Geometry: final body of the model. Coordinates: model frame, mm. A direction names the side the tool comes from. Coordinates: 2 decimals unless noted, no trailing zeros. Write each loop counter-clockwise with the first axis right and the second up, starting at its lowest first coordinate (ties: lowest second). Pieces come first, ordered by that corner, then holes.
from build123d import *

# Parameters (mm, degrees)
SKETCH1_W           = 237.236
SKETCH1_H           = 51.308
BOSS_EXTRUDE1_DEPTH = 28.829
SHELL1_T            = -1.524
FILLET1_R           = 1.905
FILLET2_R           = 1.905
SKETCH2_R           = 4.826
CUT_EXTRUDE1_DEPTH  = 2.54
SKETCH3_W           = 184.531
SKETCH3_H           = 5.08
BOSS_EXTRUDE2_DEPTH = 2.54
FILLET3_R           = 0.254


with BuildPart() as part:
    # Sketch1 → Boss-Extrude1 (new body)
    with BuildSketch(Plane.XY):
        Rectangle(SKETCH1_W, SKETCH1_H)
    extrude(amount=BOSS_EXTRUDE1_DEPTH)

    # Shell1
    shell1_openings = [part.faces().sort_by_distance(p)[0] for p in [
        (0, 0, 28.829),
    ]]
    offset(amount=SHELL1_T, openings=shell1_openings, kind=Kind.INTERSECTION)

    # Fillet1
    fillet1_edges = [part.edges().sort_by_distance(p)[0] for p in [
        (117.094, 0, 1.524),
        (117.094, -24.13, 15.1765),
        (0, 24.13, 1.524),
        (117.094, 24.13, 15.1765),
        (-117.094, 0, 1.524),
        (-117.094, 24.13, 15.1765),
        (0, -24.13, 1.524),
        (-117.094, -24.13, 15.1765),
    ]]
    fillet(fillet1_edges, radius=FILLET1_R)

    # Fillet2
    fillet2_edges = [part.edges().sort_by_distance(p)[0] for p in [
        (0, -25.654, 0),
        (-118.618, 0, 0),
        (0, 25.654, 0),
        (118.618, 0, 0),
        (118.618, -25.654, 14.4145),
        (-118.618, -25.654, 14.4145),
        (-118.618, 25.654, 14.4145),
        (118.618, 25.654, 14.4145),
    ]]
    fillet(fillet2_edges, radius=FILLET2_R)

    # Sketch2 → Cut-Extrude1 (cut)
    with BuildSketch(Plane(origin=(0, 0, 0), x_dir=(-1, 0, 0), z_dir=(0, 0, -1))):
        with Locations((-45.2, 2.46)):
            Circle(SKETCH2_R)
        with Locations((45, 2.46)):
            Circle(SKETCH2_R)
    extrude(amount=-CUT_EXTRUDE1_DEPTH, mode=Mode.SUBTRACT)

    # Sketch3 → Boss-Extrude2 (add)
    with BuildSketch(Plane(origin=(0, -24.13, 0), x_dir=(1, 0, 0), z_dir=(0, 1, 0))):
        with Locations((0, -26.289)):
            Rectangle(SKETCH3_W, SKETCH3_H)
    extrude(amount=BOSS_EXTRUDE2_DEPTH)

    # Fillet3
    fillet3_edges = [part.edges().sort_by_distance(p)[0] for p in [
        (-92.2655, -24.13, 26.289),
        (-92.2655, -22.86, 23.749),
        (92.2655, -24.13, 26.289),
        (0, -24.13, 23.749),
        (92.2655, -22.86, 23.749),
        (-92.2655, -21.59, 26.289),
        (92.2655, -21.59, 26.289),
        (0, -21.59, 23.749),
    ]]
    fillet(fillet3_edges, radius=FILLET3_R)


solid = part.part
Item 1: Pin query (flat end, axial travel): pin 1 (8.5 mm diameter, centred on x = -45, y = 2.46, fed in from +Z); pin 2 (6 mm diameter, centred on x = 54, y = 11, fed in from +Z); pin 3 (10 mm diameter, centred on x = -34.5, y = 1.5, fed in from -Z). Return the tip coordinate at first contact, or that it passes through.
Derived:
pin 1: passes through
pin 2: stops at z = 1.52
pin 3: stops at z = 0
Item 2: Set-up query: faces 1 (the flat face through (-2, -24.13, 13)), 2 (the flat face through (-2, 24.13, 16)), 3 (the cylindrical face through (50.02, 2.67, 0.75)). Return all of +Z, -Z, +X, -X, +Y, -Y with unobstructed straight access to the full face (end or side cutting, diameter ignored); none if empty.
Derived:
face 1: none
face 2: +Z
face 3: +Z, -Z
Item 3: Section D-D, the plane x = 97.5. Output: boundary loops of the cut face in (y, z) (3 decimals).
Derived:
outline: (-25.654, 1.905) arc R1.905 ccw to (-23.749, 0) - (23.749, 0) arc R1.905 ccw to (25.654, 1.905) - (25.654, 28.829) - (24.13, 28.829) - (24.13, 3.429) arc R1.905 cw to (22.225, 1.524) - (-22.225, 1.524) arc R1.905 cw to (-24.13, 3.429) - (-24.13, 28.829) - (-25.654, 28.829) - close
Item 4: Pull-direction query (Y, two-part tool) for faces 4 (the flat face through (-117.094, 0, 16)), 5 (the flat face through (-2, 0, 0)), 6 (the flat face through (-2, -25.654, 15)); classes: released by +Y, released by -Y, zero draft, split by the parting line, or undercut.
Derived:
face 4: undercut
face 5: zero draft
face 6: released by -Y
Item 5: Section B-B, the plane x = -45. Output: boundary loops of the cut face in (y, z) (3 decimals), plus the area to 3 significant figures.
Derived:
outline: (-25.654, 1.905) arc R1.905 ccw to (-23.749, 0) - (-2.366, 0) - (-2.366, 1.524) - (-22.225, 1.524) arc R1.905 cw to (-24.13, 3.429) - (-24.13, 23.495) arc R0.254 cw to (-23.876, 23.749) - (-21.844, 23.749) arc R0.254 ccw to (-21.59, 24.003) - (-21.59, 28.829) - (-25.654, 28.829) - close; (7.286, 0) - (23.749, 0) arc R1.905 ccw to (25.654, 1.905) - (25.654, 28.829) - (24.13, 28.829) - (24.13, 3.429) arc R1.905 cw to (22.225, 1.524) - (7.286, 1.524) - close
area: 160 mm2
Item 6: Section A-A, the plane y = 2.46. Output: boundary loops of the cut face in (x, z) (3 decimals), plus the area to 3 significant figures.
Derived:
outline: (-118.618, 1.905) arc R1.905 ccw to (-116.713, 0) - (-49.826, 0) - (-49.826, 1.524) - (-115.189, 1.524) arc R1.905 cw to (-117.094, 3.429) - (-117.094, 28.829) - (-118.618, 28.829) - close; (-40.174, 0) - (40.374, 0) - (40.374, 1.524) - (-40.174, 1.524) - close; (50.026, 0) - (116.713, 0) arc R1.905 ccw to (118.618, 1.905) - (118.618, 28.829) - (117.094, 28.829) - (117.094, 3.429) arc R1.905 cw to (115.189, 1.524) - (50.026, 1.524) - close
area: 415 mm2
Item 7: Material intervals for probe 1 along Y at (x, z) = (-58, 20.5); probe 2 along X at (y, z) = (-21, 8); probe 3 along Z at (x, y) = (-107.5, 5), sorted ascending.
Derived:
probe 1: y = -25.65 to -24.13, 24.13 to 25.65
probe 2: x = -118.62 to -117.09, 117.09 to 118.62
probe 3: z = 0 to 1.52
Item 8: Section C-C, the plane z = 11.75. Output: boundary loops of the cut face in (x, y) (3 decimals).
Derived:
outline: (-118.618, -23.749) arc R1.905 ccw to (-116.713, -25.654) - (116.713, -25.654) arc R1.905 ccw to (118.618, -23.749) - (118.618, 23.749) arc R1.905 ccw to (116.713, 25.654) - (-116.713, 25.654) arc R1.905 ccw to (-118.618, 23.749) - close; hole (-117.094, -22.225) arc R1.905 ccw to (-115.189, -24.13) - (115.189, -24.13) arc R1.905 ccw to (117.094, -22.225) - (117.094, 22.225) arc R1.905 ccw to (115.189, 24.13) - (-115.189, 24.13) arc R1.905 ccw to (-117.094, 22.225) - close
